Can you work these out from the model? Positions are in its coordinate system, mm. A direction names the side the tool comes from. Round coordinates to 2 decimals unless told otherwise and drop trailing zeros. Order: outer loops, then holes, each group sorted by start corner. A loop starts at its lowest first (then second) coordinate and runs counter-clockwise, first axis right, second up. Notation, with made-up numbers: M 37.25,1.25 L 86.25,1.25 A28 ccw 86.25,38.25 Z; hole C -27,68.25 d8. An arc over 180 degrees is marked long. Answer as a JSON object with one key per item and string values. Group by question number.
from build123d import *

# Parameters (mm, degrees)
F3_DEPTH = 8


with BuildPart() as f1:
    # F0 (on Front) → F1 (revolve)
    with BuildSketch(Plane.XZ):
        with BuildLine():
            ThreePointArc((17.75, -3), (18.6286796564, -0.8786796564), (20.75, 0))
            Line((20.75, 0), (26.5, 0))
            Line((26.5, 0), (26.5, 6))
            Line((26.5, 6), (23.425, 6))
            Line((23.425, 6), (23.425, 10.5))
            add(Edge.make_bspline(
                [(23.425, 10.5), (23.425, 16), (0, 16)],
                knots=[3.1415926536, 3.1415926536, 3.1415926536, 4.7123889804, 4.7123889804, 4.7123889804], degree=2, weights=[1, 0.7071067812, 1]))
            Line((0, 16), (0, 13))
            add(Edge.make_bspline(
                [(20.425, 10.1929514026), (20.425, 13), (0, 13)],
                knots=[0, 0, 0, 1.5707963268, 1.5707963268, 1.5707963268], degree=2, weights=[1, 0.7071067812, 1]))
            Line((20.425, 10.1929514026), (20.425, 5))
            Line((20.425, 5), (0, 5))
            Line((0, 5), (0, 2))
            Line((0, 2), (13.75, 2))
            ThreePointArc((13.75, 2), (14.4571067812, 1.7071067812), (14.75, 1))
            Line((14.75, 1), (14.75, -6))
            Line((14.75, -6), (17.75, -6))
            Line((17.75, -6), (17.75, -3))
        make_face()
    revolve(axis=Axis((0, 0, 3), (0, 0, 1)))

    # F2 (on face) → F3 (join, through all)
    with BuildSketch(Plane(origin=(0, 0, 2), x_dir=(1, 0, 0), z_dir=(0, 0, -1))):
        Polygon((2.8637252952, 3.9852742399), (-2.0194860852, 4.472695975), (-4.8832113804, 0.4874217352), (-2.8637252952, -3.9852742399), (2.0194860852, -4.472695975), (4.8832113804, -0.4874217352), align=None)
        Polygon((-1.5443128887, 3.4202969221), (2.1899075787, 3.047562654), (3.7342204673, -0.3727342681), (1.5443128887, -3.4202969221), (-2.1899075787, -3.047562654), (-3.7342204673, 0.3727342681), align=None, mode=Mode.SUBTRACT)
    extrude(amount=F3_DEPTH)


solid = f1.part
Item 1: On a 3-axis mill with a long thin cutter (end or side, diameter ignored), from which of +Z, -Z, +X, -X, +Y, -Y can I reach the whole of each face in a straight line? I mean faces 4 (the face through (0, 0, 5)), 5 (the face through (16, -18, 6)), 6 (the face through (-3.888, 1.718, -1.944)). Say none if no direction works.
Item 2: Suppose I cut it at A-A, the plane z = 7.25. Write out the boundary of the cut face in (x, y) (3 decimals).
Item 3: I need wall thicknesses on line 1 (Y direction, x = 0, z = 7.65) (3 decimals); line 2 (Y direction, x = -3, z = -3.5); line 3 (Z direction, x = 22, y = -10). Which ranges of each line are inside material? Lowest first, please.
Item 4: If we mould it in two halves opening along Z, with no side actions, what happens to faces 1 (the face through (-3, 15, -6)), 2 (the face through (2.65, 1.88, -1.94)), 3 (the face through (-4.43, -19.94, 7.56))? For each: +Z half, -Z half, draft (parallel to the pull), parting line (faces both ways), or undercut.
Item 5: I'm going to push flat-ended pins straight in: pin 1 Ø22 at (x, y) = (-2, -2) entering from -Z; pin 2 Ø4 at (y, z) = (-8.5, 9.5) entering from -X; pin 3 Ø1 at (y, z) = (15.5, 6) entering from +X; pin 4 Ø10 at (x, z) = (-0.5, 12) entering from +Y (3 decimals). Where does each tip first touch, or does it pass through?
Computed:
{
 "1": {"face 4": "none", "face 5": "+Z", "face 6": "-Z"},
 "2": {"outline": "C 0,0 d46.85; hole C 0,0 d40.85"},
 "3": {"line 1": "y = -23.425 to -20.425, 20.425 to 23.425", "line 2": "y = -17.49 to -14.44, -3.11 to -1.39, 1.25 to 3.68, 14.44 to 17.49", "line 3": "z = 0 to 6"},
 "4": {"face 1": "-Z half", "face 2": "draft", "face 3": "undercut"},
 "5": {"pin 1": "stops at z = -6", "pin 2": "stops at x = -22.51", "pin 3": "stops at x = 21.85", "pin 4": "stops at y = 23.425"}
}
